```python
from build123d import *

# Parameters (mm, degrees)
F4_R = 5.99999


# Not quite as in the source:
# - a fillet or chamfer is up to 0.001 mm smaller than in the source, because OpenCascade refuses the exact size


with BuildPart() as f1:
    # F0 (on Front) → F1 (revolve)
    with BuildSketch(Plane.XZ):
        with BuildLine():
            Line((0, 31), (0, 0))
            Line((0, 0), (88, 0))
            Line((88, 0), (88, 16))
            Line((88, 16), (85, 16))
            Line((85, 16), (85, 20))
            Line((85, 20), (68, 20))
            Line((68, 20), (68, 31))
            Line((68, 31), (56, 31))
            ThreePointArc((56, 31), (50, 25), (44, 31))
            Line((44, 31), (0, 31))
        make_face()
    revolve(axis=Axis((56.2561290468, 0, 0), (1, 0, 0)))

    # F2 (on Front) → F3 (revolve, cut)
    with BuildSketch(Plane.XZ):
        Polygon((0, 25), (0, 0), (88, 0), (88, 6), (30, 6), (30, 16), (22, 16), (22, 20.5), (17, 20.5), (17, 12.5), (14, 12.5), (14, 16), (1.5, 16), (1.5, 25), align=None)
    revolve(axis=Axis((-8.4188580513, 0, 0), (-1, 0, 0)), mode=Mode.SUBTRACT)

    # F4 (radius 6 in the source; OpenCascade refuses exactly that, so slightly less here)
    f4_edges = [f1.edges().sort_by_distance(p)[0] for p in [
        (0, 0, -31),
    ]]
    fillet(f4_edges, radius=F4_R)


solid = f1.part
```
Build history of the part. All positions in model axes, mm. A direction names the side the tool comes from. Coordinates: 2 decimals unless noted, no trailing zeros. Order: outer loops, then holes, each group sorted by start corner. A loop starts at its lowest first (then second) coordinate and runs counter-clockwise, first axis right, second up. Notation, with made-up numbers: (69, 87.5) -> (114, 87.5) arc R21 cw to (114, 94.5) -> close; hole circle Ø8 at (-35, 12). An arc over 180 degrees is marked (long way). Answer in a Markdown table with one row per item. Add a question column.
Q1. Wall check: line 1 along X through (y, z) = (18, 0.5); line 2 along Y through (x, z) = (15.8, 0); line 3 along Y through (x, z) = (19, 0). Give the ranges that are in metal, low to high. Write a range as [from, to].
Q2. Mould opens along Z. For faces 1 (the face through (19.465, -20.013, -4.444)), 2 (the face through (86.48, 15.62, -3.47)), 3 (the face through (85, -13.43, 8.98)) say: +Z half, -Z half, draft (parallel to the pull), parting line (faces both ways), or undercut.
Q3. Drop flat-ended pins along their axis: pin 1 (4 mm diameter, centred on x = 35.5, y = -17, fed in from -Z); pin 2 (9.5 mm diameter, centred on y = 0, z = 0, fed in from -X) (3 decimals); pin 3 (22.5 mm diameter, centred on y = 0, z = 0, fed in from -X); pin 4 (10 mm diameter, centred on x = 57, y = -7, fed in from -Z). Give the stop position or say it passes through.
Q4. Band-saw the part on A-A, the plane x = 28. List the corners of the cut face in (y, z), then the cut area to 3 significant figures.
Q5. Which spindle directions (+Z, -Z, +X, -X, +Y, -Y) get a long thin tool onto all of the face, cutting with end or side? Do faces 4 (the face through (7.66, -15.62, -3.47)), 5 (the face through (17, -9, -9)), 6 (the face through (76.381, 19.524, -4.336)). Say none if no direction does.
Answers follow:
| question | item | result |
|---|---|---|
| 1 | line 1 | [1.5, 17], [22, 85] |
| 1 | line 2 | [-31, -12.5], [12.5, 31] |
| 1 | line 3 | [-31, -20.5], [20.5, 31] |
| 2 | face 1 | undercut |
| 2 | face 2 | parting line |
| 2 | face 3 | draft |
| 3 | pin 1 | z = -27.13 |
| 3 | pin 2 | through |
| 3 | pin 3 | x = 30 |
| 3 | pin 4 | z = -30.94 |
| 4 | outline | circle Ø62 at (0, 0); hole circle Ø32 at (0, 0) |
| 4 | area | 2,210 mm^2 |
| 5 | face 4 | -X |
| 5 | face 5 | none |
| 5 | face 6 | +X |
